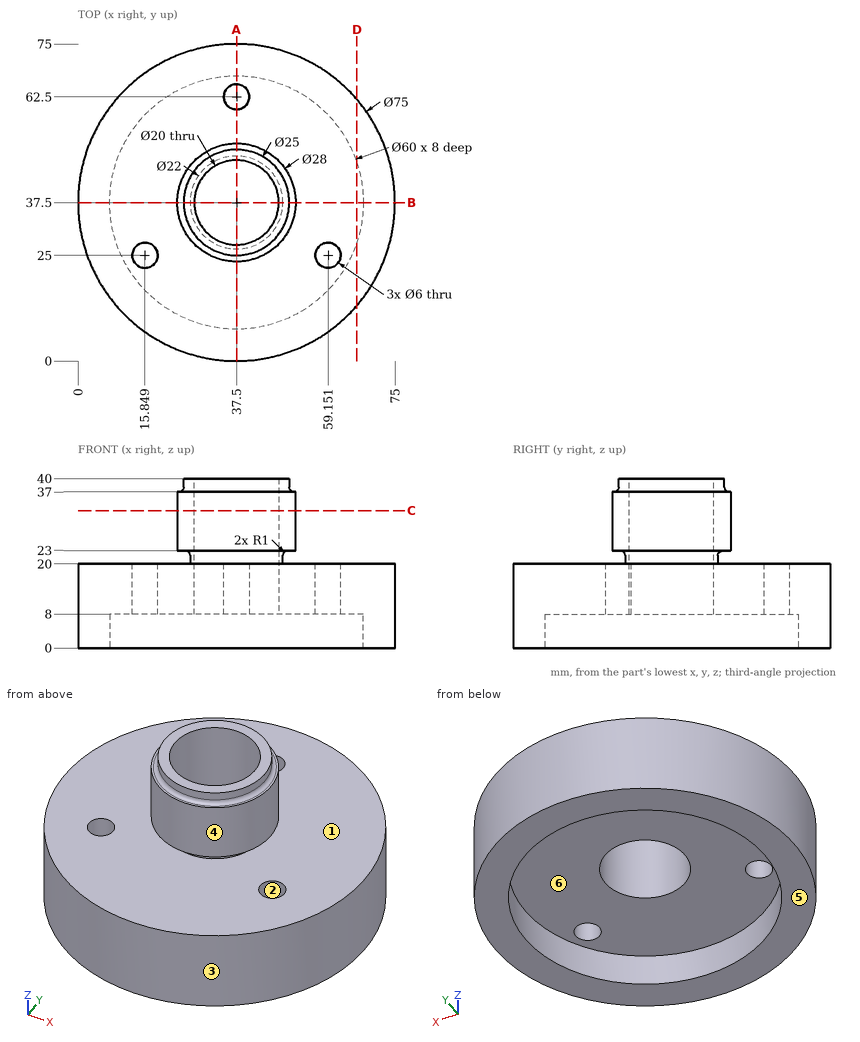
Geometry check sheet. Reference: drawing and pictorial views, mm from the part's lowest x, y, z. A direction names the side the tool comes from. Give positions to 0.01 mm unless a question says otherwise; leave off trailing zeros. Order: outer loops, then holes, each group sorted by start corner. A loop starts at its lowest first (then second) coordinate and runs counter-clockwise, first axis right, second up. Notation, with made-up numbers: (8, 12) - (58, 12) arc R15 ccw to (58, 41) - close; hole circle Ø6 at (34, -5). An arc over 180 degrees is marked (long way). Use one line per item in the form item = value.
1) Access from +Z, -Z, +X, -X, +Y, -Y to the whole of each face (thin tool, end or side, straight path). Record for the marked faces 4, 5 and 6.
Working result:
face_4 = +Z
face_5 = -Z, +X, -X, +Y, -Y
face_6 = -Z
2) Sectioned sample at C-C (z = 32.5). Record the boundary of the cut face in (x, y).
Working result:
outline = circle Ø28 at (37.5, 37.5); hole circle Ø20 at (37.5, 37.5)
3) Sectioned sample at D-D (x = 66). Record the boundary of the cut face in (y, z), and give its area (3 significant figures).
Working result:
outline = (13.13, 0) - (28.13, 0) - (28.13, 8) - (46.87, 8) - (46.87, 0) - (61.87, 0) - (61.87, 20) - (13.13, 20) - close
area = 825 mm^2
4) Draft check along Y on the marked faces 1, 2 and 3. Enter one of: released by +Y, released by -Y, zero draft, split by the parting line, or undercut.
Working result:
face_1 = zero draft
face_2 = undercut
face_3 = split by the parting line
5) Depth check by flat-ended pin: pin 1 Ø3 at (x, y) = (49.5, 14.5) entering from +Z; pin 2 Ø6 at (y, z) = (47.5, 4.5) entering from +X; pin 3 Ø10 at (x, z) = (14.5, 21) entering from +Y. Enter the tip coordinate at first touch or a pass-through.
Working result:
pin_1 = 20
pin_2 = 74.34
pin_3 = 70.34
6) Sectioned sample at A-A (x = 37.5). Count the separate pieces of the cut face and the enclosed holes in it, and give its area (3 significant figures).
Working result:
separate_pieces = 3
enclosed_holes = 0
area = 842 mm^2
7) Material ranges on probe 1 along Y at (x, z) = (37.5, 17); probe 2 along X at (y, z) = (37, 2); probe 3 along Z at (x, y) = (27, 43), recorded low to high. Write a range as from..to.
Working result:
probe_1 = 0..27.5, 47.5..59.5, 65.5..75
probe_2 = 0..7.5, 67.5..75
probe_3 = 8..20, 22.99..40
8) Sectioned sample at B-B (y = 37.5). Record the boundary of the cut face in (x, z).
Working result:
outline = (0, 0) - (7.5, 0) - (7.5, 8) - (27.5, 8) - (27.5, 40) - (25, 40) - (25, 38) arc R1 cw to (24, 37) - (23.5, 37) - (23.5, 23) - (25.5, 23) arc R1 cw to (26.5, 22) - (26.5, 20) - (0, 20) - close; (47.5, 8) - (67.5, 8) - (67.5, 0) - (75, 0) - (75, 20) - (48.5, 20) - (48.5, 22) arc R1 cw to (49.5, 23) - (51.5, 23) - (51.5, 37) - (51, 37) arc R1 cw to (50, 38) - (50, 40) - (47.5, 40) - close
